Check sheet for the drawn part. Datum: minimum x, y, z corner. Units: mm. A direction names the side the tool comes from. Coordinates: 2 decimals unless noted, no trailing zeros. Loops run counter-clockwise (first coordinate to the right, second up) from the corner with the lowest first, then second, coordinate; pieces in that order, holes last.
Q1. Access from +Z, -Z, +X, -X, +Y, -Y to the whole of each face (thin tool, end or side, straight path). Record for the marked faces 4 and 5.
Q2. Sectioned sample at C-C (y = 5.5). Enter the section's corners in (x, z) (3 decimals), then the cut area to 3 significant figures.
Q3. Sectioned sample at D-D (x = 10.5). Enter the section's corners in (y, z), then the cut area to 3 significant figures.
Q4. Material ranges on probe 1 along Z at (x, y) = (6.5, 1.5); probe 2 along Y at (x, z) = (1.5, 6); probe 3 along X at (y, z) = (3.75, 7), recorded low to high.
Q5. Go/stop test with flat-tipped pins: P1, Ø2, axis at x = 1.5, y = 1, coming from the +Z side; P2, Ø1.5, axis at x = 5.5, y = 1.5, coming from the +Z side. Record where each tip stops, or that it passes through.
Q6. Mould release check, pull along X, two halves, no side actions. Record for the marked faces 1, 2 and 3: +X half, -X half, draft (parallel to the pull), parting line (faces both ways), or undercut.
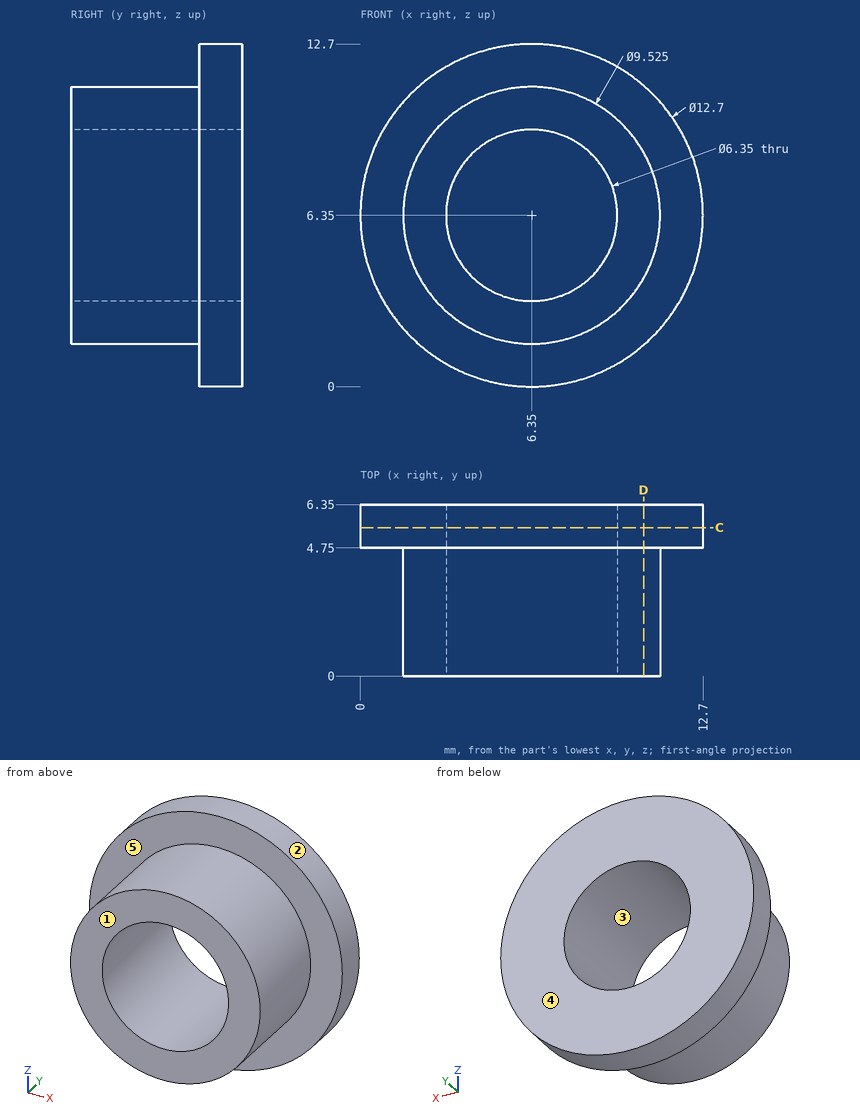
Geometry check:
1. face 4: +Z, -Z, +X, -X, +Y
1. face 5: -Y
2. outline: circle Ø12.7 at (6.35, 6.35); hole circle Ø6.35 at (6.35, 6.35)
2. area: 95.0 mm2
3. outline: (0, 4.01) - (4.75, 4.01) - (4.75, 1.54) - (6.35, 1.54) - (6.35, 11.16) - (4.75, 11.16) - (4.75, 8.69) - (0, 8.69) - close
3. area: 37.6 mm2
4. probe 1: z = 1.59 to 3.18, 9.52 to 11.11
4. probe 2: y = 4.75 to 6.35
4. probe 3: x = 1.63 to 3.24, 9.46 to 11.07
5. P1: stops at z = 9.15
5. P2: stops at z = 11.11
6. face 1: draft
6. face 2: parting line
6. face 3: undercut
